Design review of the part shown in the three views and the two pictorial views. Dimensions are in mm from the part's minimum x, y and z. A direction names the side the tool comes from. Give positions to 0.01 mm unless a question says otherwise; leave off trailing zeros. Loops run counter-clockwise (first coordinate to the right, second up) from the corner with the lowest first, then second, coordinate; pieces in that order, holes last.
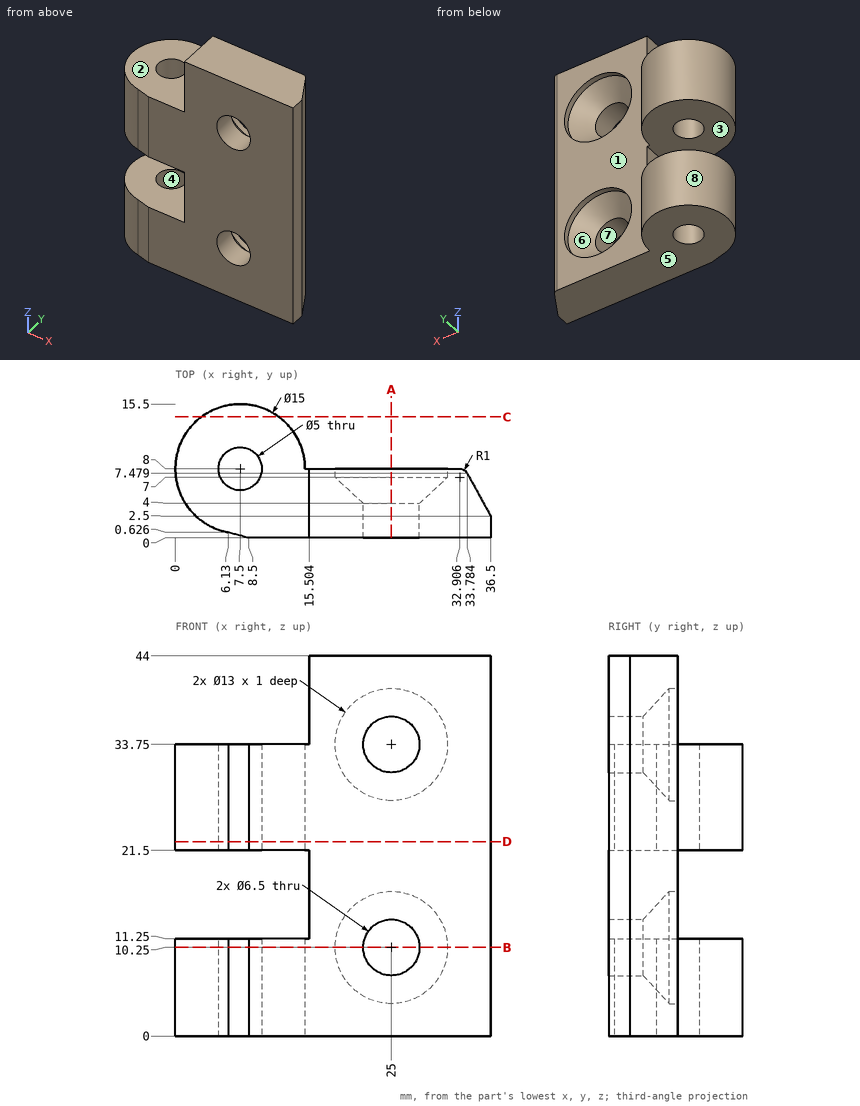
Q1. Tool access review of the marked faces 1, 2, 3 and 4: name each direction out of +Z, -Z, +X, -X, +Y, -Y from which nothing blocks a thin tool from reaching the whole face with its end or side.
Results:
face 1: +Z, -Z, +X, +Y
face 2: +Z, -X, +Y, -Y
face 3: -X, +Y, -Y
face 4: +Z, -Z
Q2. Wall thickness on line 1 (Z direction, x = 12, y = 2); line 2 (X direction, y = 7.45, z = 10.25); line 3 (Y direction, x = 18, z = 6): over which ranges is each line inside the solid? List them lowest first.
Results:
line 1: z = 0 to 11.25, 21.5 to 33.75
line 2: x = 0.02 to 5.06, 9.94 to 18.5, 31.5 to 33.8
line 3: y = 0 to 8
Q3. Insertion check: pin 1 (9 mm diameter, centred on y = 2.5, z = 15.5, fed in from -X); pin 2 (4.5 mm diameter, centred on x = 4, y = 6.5, fed in from +Z); pin 3 (4 mm diameter, centred on y = 4.5, z = 36.5, fed in from -X). Each pin has a flat end and moves straight along its axis. Give the tip position at first contact, or say it passes through.
Results:
pin 1: stops at x = 1.17
pin 2: stops at z = 33.75
pin 3: stops at x = 15.5
Q4. Take a section at C-C (y = 14). Give the boundary of the cut face in (x, z).
Results:
outline: (3, 0) - (12, 0) - (12, 11.25) - (3, 11.25) - close; (3, 21.5) - (12, 21.5) - (12, 33.75) - (3, 33.75) - close
Q5. Draft analysis for pull direction Z (two halves, no side actions). For the marked faces 5, 6, 7 and 8, state which applies: pulls with the +Z half, pulls with the -Z half, needs draft (parallel to the pull), parting line crosses it, or undercut.
Results:
face 5: pulls with the -Z half
face 6: undercut
face 7: undercut
face 8: needs draft
Q6. Take a section at A-A (x = 25). Give the boundary of the cut face in (y, z).
Results:
outline: (0, 0) - (8, 0) - (8, 3.75) - (7, 3.75) - (4, 7) - (0, 7) - close; (0, 13.5) - (4, 13.5) - (7, 16.75) - (8, 16.75) - (8, 27.25) - (7, 27.25) - (4, 30.5) - (0, 30.5) - close; (0, 37) - (4, 37) - (7, 40.25) - (8, 40.25) - (8, 44) - (0, 44) - close
Q7. Take a section at D-D (z = 22.5). Give the boundary of the cut face in (x, y) (1 decimal), plus the area to 3 significant figures.
Results:
outline: (6.1, 0.6) - (8.5, 0) - (36.5, 0) - (36.5, 2.5) - (33.8, 7.5) arc R1 ccw to (32.9, 8) - (15, 8) arc R7.5 ccw (long way) to start; hole circle Ø5 at (7.5, 8)
area: 337 mm2
Q8. Take a section at B-B (z = 10.25). Give the number of separate pieces and of enclosed holes in the cut face, plus the area to 3 significant figures.
Results:
separate pieces: 2
enclosed holes: 1
area: 268 mm2
